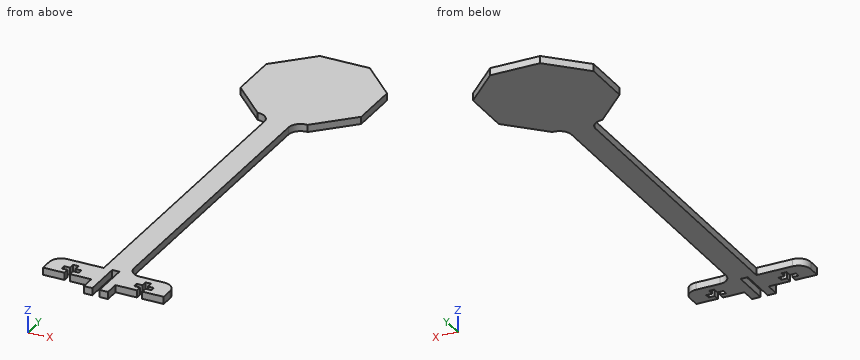
from build123d import *

# Parameters (mm, degrees)
BOSS_EXTRUDE1_DEPTH = 3
FILLET1_R           = 5


with BuildPart() as part:
    # Sketch1 → Boss-Extrude1 (new body)
    with BuildSketch(Plane.XY):
        Polygon((-5, -25), (-5, -159), (-25, -159), (-25, -169), (-16.1, -169), (-16.1, -166.5), (-18.6, -166.5), (-18.6, -164.5), (-16.1, -164.5), (-16.1, -162), (-13.9, -162), (-13.9, -164.5), (-11.4, -164.5), (-11.4, -166.5), (-13.9, -166.5), (-13.9, -169), (-5, -169), (-5, -175), (-1.5, -175), (-1.5, -159), (1.5, -159), (1.5, -175), (5, -175), (5, -169), (13.9, -169), (13.9, -166.5), (11.4, -166.5), (11.4, -164.5), (13.9, -164.5), (13.9, -162), (16.1, -162), (16.1, -164.5), (18.6, -164.5), (18.6, -166.5), (16.1, -166.5), (16.1, -169), (25, -169), (25, -159), (5, -159), (5, -25), (10.355339059, -25), (25, -10.355339059), (25, 10.355339059), (10.355339059, 25), (-10.355339059, 25), (-25, 10.355339059), (-25, -10.355339059), (-10.355339059, -25), align=None)
    extrude(amount=BOSS_EXTRUDE1_DEPTH)

    # Fillet1
    fillet1_edges = [part.edges().sort_by_distance(p)[0] for p in [
        (5, -25, 1.5),
        (5, -159, 1.5),
        (25, -159, 1.5),
        (-25, -159, 1.5),
        (-5, -25, 1.5),
    ]]
    fillet(fillet1_edges, radius=FILLET1_R)


solid = part.part
The model under review builds one solid part; all positions refer to its coordinate system, in mm. Round coordinates to 2 decimals unless told otherwise and drop trailing zeros. Write each loop counter-clockwise with the first axis right and the second up, starting at its lowest first coordinate (ties: lowest second). Pieces come first, ordered by that corner, then holes. Notation, with made-up numbers: (78.5, 54.5) - (92.5, 54.5) arc R30 ccw to (92.5, 83.5) - close; hole circle Ø10 at (19.25, 4.5). An arc over 180 degrees is marked (long way). One line per item, written item: value. Start each with the question number.
1. To check wall thickness, follow L1, parallel to Y at x = -12, z = 2.7; L2, parallel to Y at x = -18, z = 1.6; L3, parallel to X at y = -118, z = 0.75. State the ranges of each line that lie inside material, in increasing order. Write a range as from..to.
2. Consider section A-A on y = -76. Write out the cut boundary in (x, z), and give its area (3 significant figures).
3. Clearance check with flat-ended pins moving along their axes: P1, Ø6, axis at x = -0.5, y = -28.5, coming from the -Z side; P2, Ø1.5, axis at x = -9, z = 2, coming from the -Y side; P3, Ø1.2, axis at x = 12, z = 2, coming from the +Y side; P4, Ø1.1, axis at x = 14.5, z = 1.5, coming from the -Y side. State where each tip first meets the part, or that it passes through.
Checks:
1. L1: y = -169..-166.5, -164.5..-159, -23.36..23.36
1. L2: y = -169..-166.5, -164.5..-159, -17.36..17.36
1. L3: x = -5..5
2. outline: (-5, 0) - (5, 0) - (5, 3) - (-5, 3) - close
2. area: 30.0 mm^2
3. P1: stops at z = 0
3. P2: stops at y = -169
3. P3: stops at y = 23.96
3. P4: stops at y = -162
